Here's the drawing with two shaded views (mm, measured from the low corner). I have some questions. Give positions to 0.01 mm unless a question says otherwise; leave off trailing zeros. Loops run counter-clockwise (first coordinate to the right, second up) from the corner with the lowest first, then second, coordinate; pieces in that order, holes last. Notation, with made-up numbers: (41.25, 65) - (69.25, 65) arc R10 ccw to (69.25, 83) - close; hole circle Ø9 at (88.25, 40.25). An arc over 180 degrees is marked (long way). Write each question's results on one line, items separated by ' | '. Start each with the question number.
1) I want a section at D-D, the plane z = 0.5. Write out the boundary of the cut face in (x, y).
2) If we mould it in two halves opening along Y, with no side actions, what happens to the marked faces 1, 2 and 3? For each: +Y half, -Y half, draft (parallel to the pull), parting line (faces both ways), or undercut.
3) If I drill on probe 1 along Y at (x, z) = (7, 3.75); probe 2 along Y at (x, z) = (8.5, 3.25); probe 3 along X at (y, z) = (8.75, 4.25), over which ranges is the centre line in solid material (lowest first)? Write a range as [from, to].
4) I want a section at C-C, the plane z = 2.25. Write out the boundary of the cut face in (x, y), and give its area (3 significant figures).
5) I'm going to push flat-ended pins straight in: pin 1 (3 mm diameter, centred on x = 5.5, y = 6, fed in from +Z); pin 2 (1 mm diameter, centred on x = 8.5, z = 5, fed in from -Y); pin 3 (4 mm diameter, centred on y = 4.5, z = 5.5, fed in from -X); pin 4 (1.5 mm diameter, centred on x = 6, z = 3, fed in from -Y). Where does each tip first touch, or does it pass through?
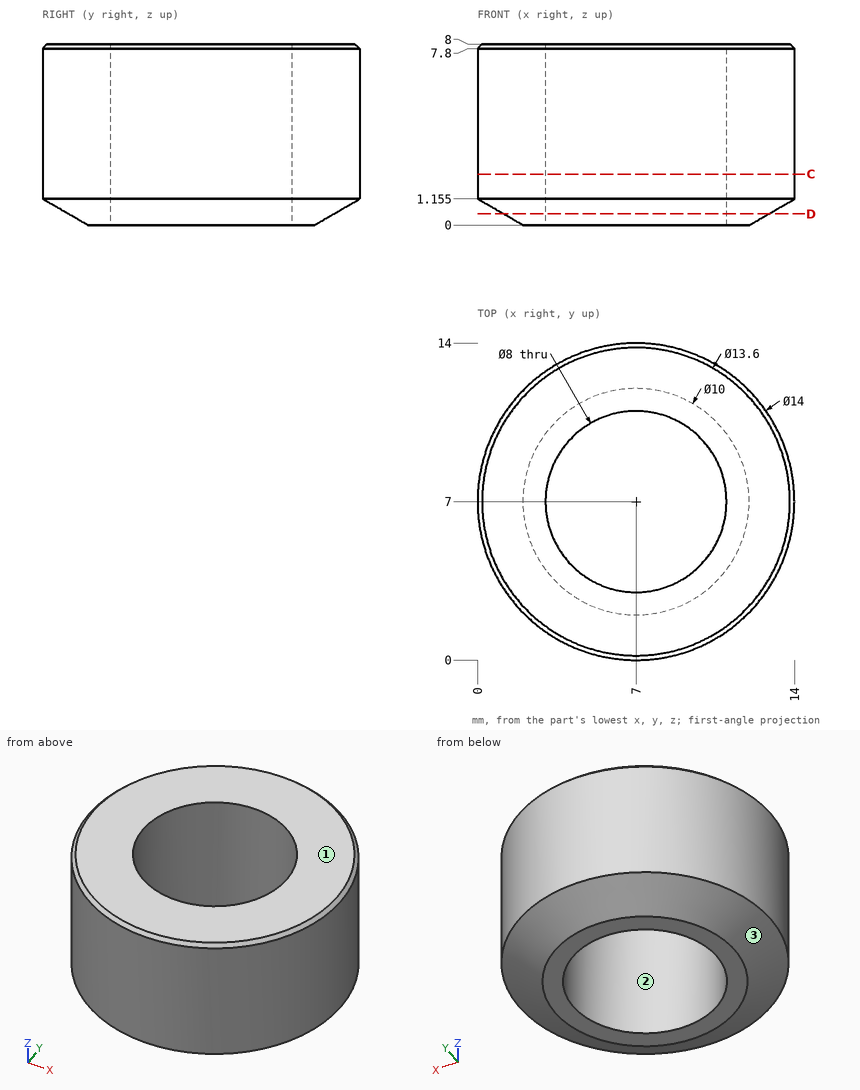
Answers:
1) outline: circle Ø11.73 at (7, 7); hole circle Ø8 at (7, 7)
2) face 1: draft | face 2: undercut | face 3: parting line
3) probe 1: y = [0, 3], [11, 14] | probe 2: y = [0.16, 3.29], [10.71, 13.84] | probe 3: x = [0.22, 3.4], [10.6, 13.78]
4) outline: circle Ø14 at (7, 7); hole circle Ø8 at (7, 7) | area: 104 mm2
5) pin 1: passes through | pin 2: stops at y = 0.07 | pin 3: stops at x = 0.02 | pin 4: stops at y = 0
